from build123d import *

# Parameters (mm, degrees)
SKETCH_1_R      = 6
EXTRUDE_1_DEPTH = 300
SKETCH_2_W      = 40
SKETCH_2_H      = 40
EXTRUDE_2_DEPTH = 225
FILLET_1_R      = 10


with BuildPart() as part:
    # 草图1 → 凸台-拉伸1 (new, symmetric)
    with BuildSketch(Plane(origin=(0, 0, 0), x_dir=(1, 0, 0), z_dir=(0, 1, 0))):
        with Locations(Location((0, 0, 0), (0, 0, 270))):
            Circle(SKETCH_1_R)
    extrude(amount=EXTRUDE_1_DEPTH, both=True)

    # 草图2 → 凸台-拉伸2 (add, symmetric)
    with BuildSketch(Plane(origin=(0, 0, 0), x_dir=(1, 0, 0), z_dir=(0, 1, 0))):
        Rectangle(SKETCH_2_W, SKETCH_2_H)
    extrude(amount=EXTRUDE_2_DEPTH, both=True)

    # 圆角1
    fillet_1_edges = [part.edges().sort_by_distance(p)[0] for p in [
        (20, 0, 20),
        (20, 0, -20),
        (-20, 0, -20),
        (-20, 0, 20),
    ]]
    fillet(fillet_1_edges, radius=FILLET_1_R)


solid = part.part
Can you work these out from the model? Positions are in its coordinate system, mm. A direction names the side the tool comes from. Coordinates: 2 decimals unless noted, no trailing zeros. Write each loop counter-clockwise with the first axis right and the second up, starting at its lowest first coordinate (ties: lowest second). Pieces come first, ordered by that corner, then holes. Notation, with made-up numbers: (23.5, 85.25) -> (62.5, 85.25) arc R28 ccw to (62.5, 106.25) -> close; hole circle Ø6 at (-23.75, 24.5). An arc over 180 degrees is marked (long way). Write each question's results on one line, items separated by ' | '. Start each with the question number.
Q1. Imagine slicing it at A-A (x = 0). Write out the boundary of the cut face in (y, z), then the cut area to 3 significant figures.
Q2. Imagine slicing it at B-B (z = 0). Write out the boundary of the cut face in (x, y).
Q3. I'm going to push flat-ended pins straight in: pin 1 (8 mm diameter, centred on x = 4.5, z = 11.5, fed in from +Y); pin 2 (2 mm diameter, centred on x = -12.5, y = 217.5, fed in from -Z); pin 3 (1.5 mm diameter, centred on y = -175, z = 11.5, fed in from +X). Where does each tip first touch, or does it pass through?
Q4. If I drill on probe 1 along Y at (x, z) = (18, 2.5); probe 2 along X at (y, z) = (-174.5, 15.5); probe 3 along Z at (x, y) = (-16.5, -168), over which ranges is the centre line in solid material (lowest first)?
Q5. Imagine slicing it at C-C (y = 212). Write out the boundary of the cut face in (x, z).
Q6. On a 3-axis mill with a long thin cutter (end or side, diameter ignored), from which of +Z, -Z, +X, -X, +Y, -Y can I reach the whole of each face in a straight line? I mean faces 1 (the face through (1.802, 263.025, 5.723)), 2 (the face through (1.802, -261.975, 5.723)), 3 (the face through (16.99, -3.15, -17.15)). Say none if no direction works.
Taken from the geometry:
1) outline: (-300, -6) -> (-225, -6) -> (-225, -20) -> (225, -20) -> (225, -6) -> (300, -6) -> (300, 6) -> (225, 6) -> (225, 20) -> (-225, 20) -> (-225, 6) -> (-300, 6) -> close | area: 19,800 mm^2
2) outline: (-20, -225) -> (-6, -225) -> (-6, -300) -> (6, -300) -> (6, -225) -> (20, -225) -> (20, 225) -> (6, 225) -> (6, 300) -> (-6, 300) -> (-6, 225) -> (-20, 225) -> close
3) pin 1: stops at y = 225 | pin 2: stops at z = -19.89 | pin 3: stops at x = 19.97
4) probe 1: y = -225 to 225 | probe 2: x = -18.35 to 18.35 | probe 3: z = -17.6 to 17.6
5) outline: (-20, -10) arc R10 ccw to (-10, -20) -> (10, -20) arc R10 ccw to (20, -10) -> (20, 10) arc R10 ccw to (10, 20) -> (-10, 20) arc R10 ccw to (-20, 10) -> close
6) face 1: +Y | face 2: -Y | face 3: -Z, +X, +Y, -Y
